Work out the finished part from the listing and answer in its coordinate system (mm). Face numbers are marked on the shaded views. A direction names the side the tool comes from. Coordinates: 2 decimals unless noted, no trailing zeros. Write each loop counter-clockwise with the first axis right and the second up, starting at its lowest first coordinate (ties: lowest second). Pieces come first, ordered by that corner, then holes. Notation, with made-up numbers: (79.5, 9.25) - (94.5, 9.25) arc R29 cw to (94.5, 45.25) - close; hole circle Ø11 at (-7, -6.5). An arc over 180 degrees is marked (long way). One line per item, written item: value.
```python
from build123d import *

# Parameters (mm, degrees)
SKETCH_1_R      = 7.5
EXTRUDE_1_DEPTH = 1.2
SKETCH_1_3_R    = 7.5
SKETCH_1_3_R_2  = 6.3
EXTRUDE_2_DEPTH = 4
SKETCH_1_5_W    = 6.2
SKETCH_1_5_H    = 6.2
EXTRUDE_3_DEPTH = 2
EXTRUDE_START   = -2
SKETCH_1_6_W    = 6.2
SKETCH_1_6_H    = 6.2
SKETCH_1_6_W_2  = 3.8
SKETCH_1_6_H_2  = 3.8
EXTRUDE_4_DEPTH = 3
FILLET_1_R      = 1
SKETCH_2_W      = 3.8
SKETCH_2_H      = 3.8
SKETCH_2_W_2    = 3.4
SKETCH_2_H_2    = 3.4
EXTRUDE_5_DEPTH = 0.8


with BuildPart() as part:
    # Эскиз1 → Бобышка-Вытянуть1 (new body)
    with BuildSketch(Plane(origin=(0, 0, 0), x_dir=(1, 0, 0), z_dir=(0, 1, 0))):
        Circle(SKETCH_1_R)
    extrude(amount=-EXTRUDE_1_DEPTH)

    # Эскиз1<3> → Бобышка-Вытянуть2 (add)
    with BuildSketch(Plane(origin=(0, 0, 0), x_dir=(1, 0, 0), z_dir=(0, 1, 0))):
        Circle(SKETCH_1_3_R)
        Circle(SKETCH_1_3_R_2, mode=Mode.SUBTRACT)
    extrude(amount=-EXTRUDE_2_DEPTH)

    # Эскиз1<5> → Бобышка-Вытянуть3 (add)
    with BuildSketch(Plane(origin=(0, 0, 0), x_dir=(1, 0, 0), z_dir=(0, 1, 0))):
        Rectangle(SKETCH_1_5_W, SKETCH_1_5_H)
    extrude(amount=-EXTRUDE_3_DEPTH)

    # Эскиз1<6> → Бобышка-Вытянуть4 (add)
    with BuildSketch(Plane(origin=(0, 0, 0), x_dir=(1, 0, 0), z_dir=(0, 1, 0)).offset(EXTRUDE_START)):
        Rectangle(SKETCH_1_6_W, SKETCH_1_6_H)
        Rectangle(SKETCH_1_6_W_2, SKETCH_1_6_H_2, mode=Mode.SUBTRACT)
    extrude(amount=-EXTRUDE_4_DEPTH)

    # Скругление1
    fillet_1_edges = [part.edges().sort_by_distance(p)[0] for p in [
        (-7.5, 0, 0),
        (-7.5, -4, 0),
    ]]
    fillet(fillet_1_edges, radius=FILLET_1_R)

    # Эскиз2 → Бобышка-Вытянуть5 (add)
    with BuildSketch(Plane.XZ.offset(5)):
        Rectangle(SKETCH_2_W, SKETCH_2_H)
        Rectangle(SKETCH_2_W_2, SKETCH_2_H_2, mode=Mode.SUBTRACT)
    extrude(amount=-EXTRUDE_5_DEPTH)


solid = part.part
```
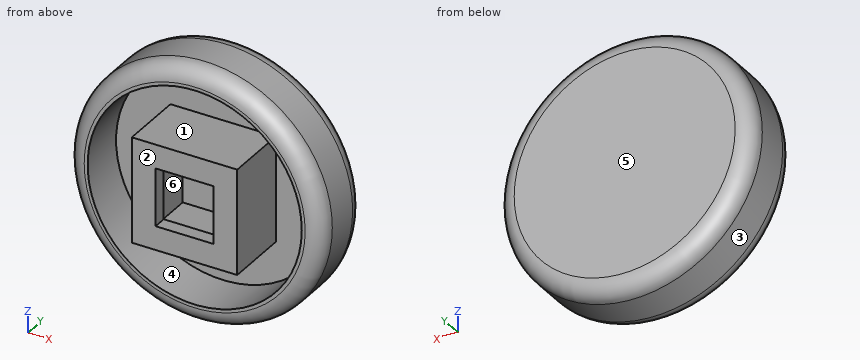
Item 1: Determine the mould class of the marked faces 1, 2 and 3 for opening direction Z: +Z half, -Z half, draft (parallel to the pull), parting line (faces both ways), or undercut.
Evaluation:
face 1: undercut
face 2: draft
face 3: parting line
Item 2: Section D-D, the plane x = 0 is taken. Determine the outline of the cut face in (y, z).
Evaluation:
outline: (-5, -3.1) - (-1.2, -3.1) - (-1.2, -6.3) - (-4, -6.3) - (-4, -6.5) arc R1 ccw to (-3, -7.5) - (-1, -7.5) arc R1 ccw to (0, -6.5) - (0, 6.5) arc R1 ccw to (-1, 7.5) - (-3, 7.5) arc R1 ccw to (-4, 6.5) - (-4, 6.3) - (-1.2, 6.3) - (-1.2, 3.1) - (-5, 3.1) - (-5, 1.7) - (-4.2, 1.7) - (-4.2, 1.9) - (-2, 1.9) - (-2, -1.9) - (-4.2, -1.9) - (-4.2, -1.7) - (-5, -1.7) - close
Item 3: Section B-B, the plane z = 0 is taken. Determine the outline of the cut face in (x, y), then the cut area to 3 significant figures.
Evaluation:
outline: (-7.5, -3) arc R1 ccw to (-6.5, -4) - (-6.3, -4) - (-6.3, -1.2) - (-3.1, -1.2) - (-3.1, -5) - (-1.7, -5) - (-1.7, -4.2) - (-1.9, -4.2) - (-1.9, -2) - (1.9, -2) - (1.9, -4.2) - (1.7, -4.2) - (1.7, -5) - (3.1, -5) - (3.1, -1.2) - (6.3, -1.2) - (6.3, -4) - (6.5, -4) arc R1 ccw to (7.5, -3) - (7.5, -1) arc R1 ccw to (6.5, 0) - (-6.5, 0) arc R1 ccw to (-7.5, -1) - close
area: 36.3 mm2
Item 4: Section C-C, the plane y = -4.5 is taken. Determine the outline of the cut face in (x, z).
Evaluation:
outline: (-3.1, -3.1) - (3.1, -3.1) - (3.1, 3.1) - (-3.1, 3.1) - close; hole (-1.7, -1.7) - (1.7, -1.7) - (1.7, 1.7) - (-1.7, 1.7) - close
Item 5: Section A-A, the plane y = -3.45 is taken. Determine the outline of the cut face in (x, z).
Evaluation:
outline: circle Ø14.79 at (0, 0); (-3.1, -3.1) - (3.1, -3.1) - (3.1, 3.1) - (-3.1, 3.1) - close; hole circle Ø12.6 at (0, 0); hole (-1.9, -1.9) - (1.9, -1.9) - (1.9, 1.9) - (-1.9, 1.9) - close
Item 6: Given pin 1 (1.9 mm diameter, centred on y = -3.5, z = -1, fed in from +X); pin 2 (0.6 mm diameter, centred on x = -0.5, y = -5, fed in from +Z); pin 3 (2 mm diameter, centred on y = -2.5, z = 5, fed in from +X), each flat-ended and moving along its own axis, determine where each tip first touches the part or whether it passes through.
Evaluation:
pin 1: stops at x = 7.5
pin 2: stops at z = 3.1
pin 3: stops at x = 6.34
Item 7: Consider probe 1 along X at (y, z) = (-2.6, 0); probe 2 along Z at (x, y) = (0, -1.8). Determine where each line is inside the solid, lowest interval first.
Evaluation:
probe 1: x = -7.5 to -6.3, -3.1 to -1.9, 1.9 to 3.1, 6.3 to 7.5
probe 2: z = -7.5 to -6.3, -3.1 to 3.1, 6.3 to 7.5
Item 8: Which of the six approach directions +Z, -Z, +X, -X, +Y, -Y give full straight-line access (tool end or side, diameter ignored) to the marked faces 4, 5 and 6?
Evaluation:
face 4: -Y
face 5: +Z, -Z, +X, -X, +Y
face 6: none
